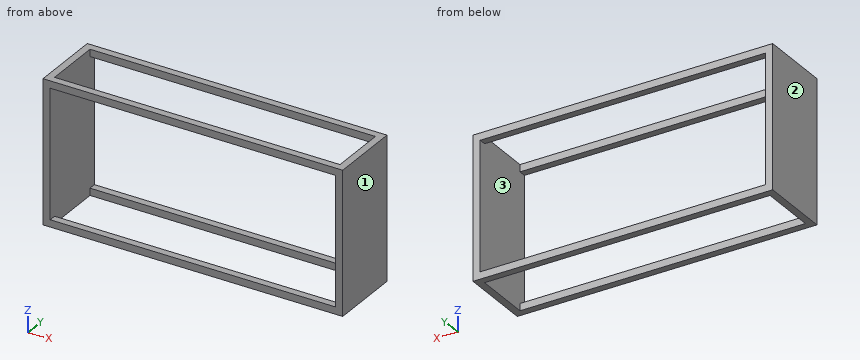
```python
from build123d import *

# Parameters (mm, degrees)
SKETCH1_W           = 2100
SKETCH1_H           = 1000
BOSS_EXTRUDE1_DEPTH = 250
CUT_EXTRUDE1_REACH  = 502
SKETCH2_W           = 2000
SKETCH2_H           = 900
SKETCH3_W           = 2000
SKETCH3_H           = 400
CUT_EXTRUDE2_DEPTH  = 1206


with BuildPart() as part:
    # Sketch1 → Boss-Extrude1 (new body, symmetric)
    with BuildSketch(Plane(origin=(0, 0, 0), x_dir=(1, 0, 0), z_dir=(0, 1, 0))):
        Rectangle(SKETCH1_W, SKETCH1_H)
    extrude(amount=BOSS_EXTRUDE1_DEPTH, both=True)

    # Sketch2 → Cut-Extrude1 (cut, up to next)
    with BuildSketch(Plane(origin=(0, 250, 0), x_dir=(1, 0, 0), z_dir=(0, 1, 0)), mode=Mode.PRIVATE) as cut_extrude1_sk1:
        Rectangle(SKETCH2_W, SKETCH2_H)
    cut_extrude1_tool1 = extrude(cut_extrude1_sk1.sketch, amount=-CUT_EXTRUDE1_REACH, mode=Mode.PRIVATE) & part.part
    add(cut_extrude1_tool1.solids().sort_by_distance((0, 250, 0))[0], mode=Mode.SUBTRACT)

    # Sketch3 → Cut-Extrude2 (cut)
    with BuildSketch(Plane(origin=(0, 0, -500), x_dir=(-1, 0, 0), z_dir=(0, 0, -1))):
        Rectangle(SKETCH3_W, SKETCH3_H)
    extrude(amount=-CUT_EXTRUDE2_DEPTH, mode=Mode.SUBTRACT)


solid = part.part
```
Verification items for the finished model (mm, model axes). Face numbers are marked on the shaded views. Give positions to 0.01 mm unless a question says otherwise; leave off trailing zeros. Loops run counter-clockwise (first coordinate to the right, second up) from the corner with the lowest first, then second, coordinate; pieces in that order, holes last. Notation, with made-up numbers: M 3,1 L 48,1 A20 ccw 48,39 Z; hole C 17,44.5 d8. An arc over 180 degrees is marked long. Return JSON: item names as keys, results as strings.
1) Section check A-A, the plane y = 115.5. Enter the section's corners in (x, z).
Findings:
{"outline": "M -1050,-500 L -1000,-500 L -1000,500 L -1050,500 Z; M 1000,-500 L 1050,-500 L 1050,500 L 1000,500 Z"}
2) Section check B-B, the plane x = -425. Enter the section's corners in (y, z).
Findings:
{"outline": "M -250,-500 L -200,-500 L -200,-450 L -250,-450 Z; M -250,450 L -200,450 L -200,500 L -250,500 Z; M 200,-500 L 250,-500 L 250,-450 L 200,-450 Z; M 200,450 L 250,450 L 250,500 L 200,500 Z"}
3) Section check C-C, the plane z = 101.5. Enter the section's corners in (x, y), and give its area (3 significant figures).
Findings:
{"outline": "M -1050,-250 L -1000,-250 L -1000,250 L -1050,250 Z; M 1000,-250 L 1050,-250 L 1050,250 L 1000,250 Z", "area": "50,000 mm2"}
4) Mould release check, pull along X, two halves, no side actions. Record for the marked faces 1, 2 and 3: released by +X, released by -X, zero draft, split by the parting line, or undercut.
Findings:
{"face 1": "released by +X", "face 2": "released by -X", "face 3": "undercut"}
5) Material ranges on L1, parallel to X at y = 108, z = 216, recorded low to high. Write a range as [from, to].
Findings:
{"L1": "x = [-1050, -1000], [1000, 1050]"}
